Autodesk Inventor part; units mm, degrees
ref_plane "YZ Plane" through (0, 0, 0) normal (1, 0, 0) x (0, 1, 0)
ref_plane "XZ Plane" through (0, 0, 0) normal (0, 1, 0) x (-1, 0, 0)
ref_plane "XY Plane" through (0, 0, 0) normal (0, 0, 1) x (1, 0, 0)
sketch "Sketch1" plane through (0, 0, 0) normal (0, 1, 0) x (-1, 0, 0)
  line L0 (63.5, 88.9) -> (-63.5, 88.9)
  line L1 (-63.5, 88.9) -> (-63.5, -88.9)
  line L2 (-63.5, -88.9) -> (63.5, -88.9)
  line L3 (63.5, -88.9) -> (63.5, 88.9)
  line L4 (63.5, 88.9) -> (-63.5, -88.9) construction
  line L5 (-63.5, 88.9) -> (63.5, -88.9) construction
  point P0 (0, 0)
  dimension "d0" = 177.8
  dimension "d1" = 127
extrude "main chassis frame" add sketch "Sketch1" along normal blind 6.35
sketch "Sketch4" plane through (0, 6.35, 0) normal (0, 1, 0) x (1, 0, 0)
  circle A0 centre (54.8311, -78.0654) radius 2.3812
  circle A1 centre (54.8311, -43.3944) radius 2.3812
  line L0 (54.8311, -75.6842) -> (54.8311, -45.7757) construction
  circle A2 centre (26.4212, -78.0654) radius 2.3812
  circle A3 centre (26.4212, -43.3944) radius 2.3812
  line L1 (26.4212, -75.6842) -> (26.4212, -45.7757) construction
  line L2 (28.8024, -78.0654) -> (52.4498, -78.0654) construction
  point P0 (0, 0)
  dimension "d19" = 4.7625
  dimension "d165" = 4.7625
  dimension "d164" = 29.9085
  dimension "d166" = 29.9085
  dimension "d167" = 23.6474
extrude "mounting holes for caster" cut sketch "Sketch4" against normal blind 6.35
sketch "Sketch5" plane through (0, 6.35, 0) normal (0, 1, 0) x (1, 0, 0)
  line L0 (63.5, 88.9) -> (-63.5, 88.9)
  line L1 (-63.5, -88.9) -> (63.5, -88.9)
  line L2 (0, 88.9) -> (-63.5, 88.9)
  line L3 (-63.5, 88.9) -> (-63.5, -88.9)
  line L4 (-63.5, -88.9) -> (0, -88.9)
  line L5 (0, -88.9) -> (0, 88.9)
  point P0 (0, 0)
  point P1 (-63.5, 88.9)
extrude "cut in half to mirror holes later" cut sketch "Sketch5" against normal blind 6.35
sketch "Sketch6" plane through (0, 0, 0) normal (0, -1, 0) x (1, 0, 0)
  circle A0 centre (19.05, -72.3766) radius 3.175
  line L0 (63.5378, -72.3766) -> (19.0878, -72.3766) construction
  line L1 (19.0878, -72.3766) -> (19.0878, -41.8966) construction
  circle A1 centre (19.0878, -41.8966) radius 3.175
  point P0 (0, 0)
  dimension "d26" = 44.45
  dimension "d27" = 6.35
  dimension "d28" = 30.48
  dimension "d29" = 6.35
extrude "zip tie mounting holes for motors" cut sketch "Sketch6" against normal blind 6.35
sketch "Sketch12" plane through (0, 6.35, 0) normal (0, 1, 0) x (1, 0, 0)
  line L0 (63.5, 88.9) -> (0, 88.9)
  line L1 (63.5, 88.9) -> (38.1, 88.9)
  line L2 (38.1, 88.9) -> (38.1, 38.1)
  line L3 (38.1, 38.1) -> (63.5, 38.1)
  line L4 (63.5, 38.1) -> (63.5, 88.9)
  point P0 (0, 0)
  dimension "d227" = 50.8
  dimension "d228" = 25.4
extrude "motor mount covers" add sketch "Sketch12" along normal blind 11.43
chamfer "motor mount slants" distance 11.1125 angle 45 1 edges at (38.1, 17.78, -63.5)
mirror "Mirror6" about plane through (0, 0, 0) normal (1, 0, 0)
sketch "Sketch22" plane through (0, 6.35, 0) normal (0, 1, 0) x (1, 0, 0)
  circle A0 centre (0, 30.1625) radius 6.35
  point P0 (0, 0)
extrude "new hole for motor wires" cut sketch "Sketch22" against normal blind 6.35
sketch "arduino uno mounting holes" plane through (0, 6.35, 0) normal (0, 1, 0) x (1, 0, 0)
  line L0 (-63.5, -88.9) -> (-63.5, 88.9)
  line L1 (-58.42, -17.7229) -> (-58.42, 33.0771) construction
  circle A0 centre (-46.0375, 29.5275) radius 1.778
  circle A1 centre (-47.3075, -18.7325) radius 1.778
  circle A2 centre (4.7625, 14.2875) radius 1.778
  circle A3 centre (4.7625, -13.6525) radius 1.778
  line L2 (-46.0375, 34.2699) -> (-46.0375, -23.7548) construction
  line L3 (-47.3075, -22.4854) -> (-47.3075, 33.7972) construction
  line L4 (4.7625, -21.8575) -> (4.7625, 22.1977) construction
  line L5 (15.8332, 14.2875) -> (-15.1882, 14.2875) construction
  line L6 (-52.07, 29.5275) -> (-2.2478, 29.5275) construction
  line L7 (11.43, -13.6525) -> (-14.3019, -13.6525) construction
  line L8 (-51.7639, -18.7325) -> (-2.8575, -18.7325) construction
  point P0 (0, 0)
  dimension "d186" = 3.556
  dimension "d219" = 1.27
  dimension "d220" = 15.24
  dimension "d221" = 27.94
  dimension "d222" = 5.08
  dimension "d223" = 50.8
extrude "uno mounting holes" cut sketch "arduino uno mounting holes" against normal blind 6.35
sketch "motor mount holes sketch" plane through (0, 6.35, 0) normal (0, 1, 0) x (1, 0, 0)
  line L0 (12.2391, 24.4663) -> (55.7366, 24.4663) construction
  line L1 (55.7366, 24.4663) -> (55.7366, -19.0312) construction
  line L2 (55.7366, -19.0312) -> (12.2391, -19.0312) construction
  line L3 (12.2391, -19.0312) -> (12.2391, 24.4663) construction
  circle A0 centre (52.0566, 20.7844) radius 1.778
  line L4 (52.1191, 22.5613) -> (52.1191, 24.4663) construction
  line L5 (53.8316, 20.8881) -> (55.7366, 20.8881) construction
  circle A1 centre (14.5948, 20.8847) radius 1.778
  line L6 (16.206, 21.6364) -> (50.496, 21.6364) construction
  circle A2 centre (52.1171, -16.6794) radius 1.778
  line L7 (52.888, -15.0773) -> (52.888, 19.2127) construction
  circle A3 centre (14.6521, -16.6794) radius 1.778
  line L8 (16.2396, -15.8787) -> (50.5296, -15.8787) construction
  point P0 (0, 0)
  dimension "d224" = 3.556
  dimension "d208" = 43.4975
  dimension "d209" = 43.4975
  dimension "d210" = 1.905
  dimension "d211" = 1.905
  dimension "d214" = 34.29
  dimension "d215" = 34.29
  dimension "d216" = 34.29
extrude "L298N mount holes" cut sketch "motor mount holes sketch" against normal blind 6.6675
sketch "Sketch33" plane through (0, 6.35, 0) normal (0, 1, 0) x (1, 0, 0)
  line L0 (-45.72, -25.4) -> (45.72, -25.4)
  line L1 (45.72, -25.4) -> (45.72, -88.9)
  line L2 (45.72, -88.9) -> (-45.72, -88.9)
  line L3 (-45.72, -88.9) -> (-45.72, -25.4)
  line L4 (-39.37, -31.75) -> (39.37, -31.75)
  line L5 (39.37, -31.75) -> (39.37, -82.55)
  line L6 (39.37, -82.55) -> (-39.37, -82.55)
  line L7 (-39.37, -82.55) -> (-39.37, -31.75)
  line L8 (-45.72, -60.325) -> (-63.5, -60.325) construction
  line L9 (-63.5, -88.9) -> (-63.5, 88.9)
  line L10 (45.72, -65.0875) -> (63.5, -65.0875) construction
  line L11 (63.5, -88.9) -> (63.5, 88.9)
  line L12 (-63.5, -88.9) -> (63.5, -88.9)
  point P0 (0, 0)
  dimension "d235" = 63.5
  dimension "d236" = 50.8
  dimension "d237" = 91.44
  dimension "d238" = 78.74
  dimension "d239" = 6.35
  dimension "d240" = 6.35
  dimension "d241" = 6.35
  dimension "d242" = 6.35
extrude "battery walls" add sketch "Sketch33" along normal blind 12.7
sketch "Sketch34" plane through (0, 6.35, 0) normal (0, 1, 0) x (1, 0, 0)
  line L0 (39.37, -31.75) -> (-39.37, -31.75)
  line L1 (-39.37, -82.55) -> (39.37, -82.55)
  line L2 (-31.75, -31.75) -> (-39.37, -31.75)
  line L3 (-39.37, -31.75) -> (-39.37, -82.55)
  line L4 (-39.37, -82.55) -> (-31.75, -82.55)
  line L5 (-31.75, -82.55) -> (-31.75, -31.75)
  line L6 (39.37, -82.55) -> (39.37, -31.75)
  line L7 (39.37, -31.75) -> (31.75, -31.75)
  line L8 (31.75, -31.75) -> (31.75, -82.55)
  line L9 (31.75, -82.55) -> (39.37, -82.55)
  line L10 (39.37, -82.55) -> (39.37, -31.75)
  line L11 (4.7625, -31.75) -> (-4.7625, -31.75)
  line L12 (-4.7625, -31.75) -> (-4.7625, -82.55)
  line L13 (-4.7625, -82.55) -> (4.7625, -82.55)
  line L14 (4.7625, -82.55) -> (4.7625, -31.75)
  point P0 (0, 0)
extrude "battery inner walls" add sketch "Sketch34" along normal blind 6.35 contours L6 L1 L8 L0 | L14 L1 L12 L0 | L5 L1 L3 L0
sketch "Sketch32" plane through (63.5, 0, 88.9) normal (1, 0, 0) x (0, 0, -1)
  line L0 (171.196, 6.35) -> (131.826, 6.35)
  line L1 (131.826, 6.35) -> (131.826, 13.97)
  line L2 (131.826, 13.97) -> (171.196, 13.97)
  line L3 (171.196, 13.97) -> (171.196, 6.35)
  line L4 (171.196, 10.16) -> (177.8, 10.16) construction
  line L5 (177.8, 0) -> (177.8, 17.78)
  line L6 (131.826, 9.8881) -> (127, 9.8881) construction
  line L7 (127, 6.35) -> (127, 17.78)
  line L8 (0, 6.35) -> (127, 6.35)
  point P0 (88.9, 0)
  dimension "d225" = 39.37
  dimension "d226" = 7.62
  dimension "d268" = 6.604
extrude "motor mount slot - R" cut sketch "Sketch32" against normal blind 12.7
sketch "Sketch36" plane through (0, 6.35, 0) normal (0, 1, 0) x (1, 0, 0)
  line L0 (45.72, -88.9) -> (45.72, -25.4)
  line L1 (63.5, -88.9) -> (63.5, 88.9)
  line L2 (45.72, -69.85) -> (63.5, -69.85)
  line L3 (63.5, -69.85) -> (63.5, -50.9759)
  line L4 (63.5, -50.9759) -> (45.72, -50.9759)
  line L5 (45.72, -50.9759) -> (45.72, -69.85)
  point P0 (0, 0)
extrude "side panel mount pillar" add sketch "Sketch36" along normal blind 31.75
chamfer "side panel mount pillar slant" distance 17.4625 angle 45 1 edges at (45.72, 38.1, 60.4129)
sketch "side panel mount hole" plane through (63.5, 0, 88.9) normal (1, 0, 0) x (0, 0, -1)
  circle A0 centre (28.4871, 31.0499) radius 2.3812
  line L0 (28.4871, 31.0499) -> (19.05, 31.0499) construction
  line L1 (19.05, 6.35) -> (19.05, 38.1)
  line L2 (28.4871, 31.0499) -> (37.9241, 31.0499) construction
  line L3 (37.9241, 6.35) -> (37.9241, 38.1)
  circle A1 centre (28.4871, 31.0499) radius 3.175
  point P0 (88.9, 0)
  dimension "d256" = 4.7625
  dimension "d257" = 6.35
extrude "side panel mount pillar hole - R" cut sketch "side panel mount hole" against normal blind 14.2875 contours A0 | A1
extrude "side panel mount pillar hole rim - R" add sketch "side panel mount hole" against normal blind 1.016
sketch "Sketch38" plane through (45.72, 6.35, 69.85) normal (0, 0, 1) x (1, 0, 0)
  line L0 (17.78, 0) -> (17.78, 11.43)
  line L1 (17.78, 11.43) -> (11.43, 0)
  line L2 (17.78, 0) -> (5.08, 0)
  point P0 (-45.72, -6.35)
extrude "side panel mount pillar wire passageway - R" cut sketch "Sketch38" against normal blind 19.6215
mirror "Mirror7" about plane through (0, 0, 0) normal (1, 0, 0) of "motor mount slot - R", "side panel mount pillar", "side panel mount pillar slant", "side panel mount pillar hole - R", "side panel mount pillar hole rim - R", "side panel mount pillar wire passageway - R"
sketch "side panel hole dimensions" plane through (63.5, 0, 88.9) normal (1, 0, 0) x (0, 0, -1)
  line L0 (0, 0) -> (0, 6.35)
  line L1 (19.05, 17.78) -> (19.05, 38.1)
  circle A0 centre (28.4871, 31.0499) radius 2.3812
  line L2 (177.8, 0) -> (177.8, 17.78)
  point P0 (88.9, 0)
  dimension "d264" = 19.05
  dimension "d265" = 9.4371
  dimension "d266" = 28.4871
  dimension "d267" = 149.3129
properties part number "chassis" material "Plastic, Opaque White"
Geometry: final body of the model. Coordinates: model frame, mm. A direction names the side the tool comes from. Give positions to 0.01 mm unless a question says otherwise; leave off trailing zeros. Order: outer loops, then holes, each group sorted by start corner. A loop starts at its lowest first (then second) coordinate and runs counter-clockwise, first axis right, second up. Notation, with made-up numbers: (1, 63.25) -> (60, 63.25) arc R38 ccw to (60, 102.25) -> close; hole circle Ø2 at (84.5, 47). An arc over 180 degrees is marked (long way). Answer as a JSON object with one key per item and string values.
Q1. Material intervals for probe 1 along X at (y, z) = (9.5, 75); probe 2 along Z at (x, y) = (-15.5, 12); probe 3 along X at (y, z) = (14, 27), sorted ascending.
Entries:
{"probe 1": "x = -45.72 to -31.75, -4.76 to 4.76, 31.75 to 45.72", "probe 2": "z = 25.4 to 31.75, 82.55 to 88.9", "probe 3": "x = -45.72 to 45.72"}
Q2. Section B-B (x = -19.05). Output: boundary loops of the cut face in (y, z), plus the area to 3 significant figures.
Entries:
{"outline": "(0, -88.9) -> (6.35, -88.9) -> (6.35, -75.55) -> (0, -75.55) -> close; (0, -69.2) -> (6.35, -69.2) -> (6.35, -45.07) -> (0, -45.07) -> close; (0, -38.72) -> (6.35, -38.72) -> (6.35, 25.4) -> (19.05, 25.4) -> (19.05, 31.75) -> (6.35, 31.75) -> (6.35, 82.55) -> (19.05, 82.55) -> (19.05, 88.9) -> (0, 88.9) -> close", "area": "1,210 mm^2"}
Q3. Draft query along X for faces 1 (the cylindrical face through (-45.665, 3.219, 19.413)), 2 (the flat face through (-63.5, 5, -21)), 3 (the flat face through (57, 6.35, -63)). Return one class per face: released by +X, released by -X, zero draft, split by the parting line, or undercut.
Entries:
{"face 1": "undercut", "face 2": "released by -X", "face 3": "zero draft"}
Q4. Section A-A (x = 0). Output: boundary loops of the cut face in (y, z).
Entries:
{"outline": "(0, -88.9) -> (6.35, -88.9) -> (6.35, -36.51) -> (0, -36.51) -> close; (0, -23.81) -> (6.35, -23.81) -> (6.35, 25.4) -> (19.05, 25.4) -> (19.05, 31.75) -> (12.7, 31.75) -> (12.7, 82.55) -> (19.05, 82.55) -> (19.05, 88.9) -> (0, 88.9) -> close"}
Q5. Section D-D (z = 37). Output: boundary loops of the cut face in (x, y).
Entries:
{"outline": "(-63.5, 0) -> (63.5, 0) -> (63.5, 6.35) -> (45.72, 6.35) -> (45.72, 19.05) -> (39.37, 19.05) -> (39.37, 12.7) -> (31.75, 12.7) -> (31.75, 6.35) -> (4.76, 6.35) -> (4.76, 12.7) -> (-4.76, 12.7) -> (-4.76, 6.35) -> (-31.75, 6.35) -> (-31.75, 12.7) -> (-39.37, 12.7) -> (-39.37, 19.05) -> (-45.72, 19.05) -> (-45.72, 6.35) -> (-63.5, 6.35) -> close"}
Q6. First-contact query: pin 1 (4 mm diameter, centred on x = -38, z = -27, fed in from +Y); pin 2 (10 mm diameter, centred on y = 14.5, z = 39.5, fed in from +X); pin 3 (4.5 mm diameter, centred on x = -55.5, z = -58, fed in from +Y). Flat tips, straight axial feed; report the tip coordinate or a pass-through.
Entries:
{"pin 1": "stops at y = 6.35", "pin 2": "stops at x = 45.72", "pin 3": "stops at y = 17.78"}
Q7. Section C-C (y = 25.5). Output: boundary loops of the cut face in (x, z), plus the area to 3 significant figures.
Entries:
{"outline": "(-63.5, 50.98) -> (-50.58, 50.98) -> (-50.58, 69.85) -> (-63.5, 69.85) -> close; (50.58, 50.98) -> (63.5, 50.98) -> (63.5, 69.85) -> (50.58, 69.85) -> close", "area": "488 mm^2"}
Q8. Access query for faces 4 (the cylindrical face through (4.38, 3.22, -12.55)), 5 (the flat face through (-57, 13.97, -63)), 6 (the flat face through (43.58, 12.15, -63.86)), 7 (the flat face through (-1, 14, 31.75)), 8 (the flat face through (57, 10, -42.926)). Directions: +Z, -Z, +X, -X, +Y, -Y. A direction counts if a zero-diameter tool reaches every point of the face in a straight line with its end or side. Return the directions, or none.
Entries:
{"face 4": "+Y, -Y", "face 5": "-X", "face 6": "-Z, +Y", "face 7": "+Y", "face 8": "+X"}
